Answer from the drawing. Dimensions are ordinates in mm from the lowest x, y and z of the part. Give positions to 0.01 mm unless a question says otherwise; leave off trailing zeros. Write each loop counter-clockwise with the first axis right and the second up, starting at its lowest first coordinate (ties: lowest second). Pieces come first, ordered by that corner, then holes. Notation, with made-up numbers: (76.5, -27.75) -> (132.5, -27.75) arc R30 cw to (132.5, 8.25) -> close; hole circle Ø4 at (-11.75, 70.25). An arc over 180 degrees is marked (long way). Use a Markdown table: item, result. Add a question column.
Q1. Consider line 1 (Y direction, x = 125.5, z = 1.05) (3 decimals); line 2 (X direction, y = 57, z = 2.9) (3 decimals). Determine where each line is inside the solid, lowest interval first.
Q2. Each of these flat-tipped pins is pushed along its axis until it touches: pin 1 Ø1 at (x, z) = (82, 2) entering from -Y (3 decimals); pin 2 Ø1 at (x, z) = (42.5, 1) entering from +Y; pin 3 Ø1 at (y, z) = (61, 2.5) entering from -X (3 decimals). Where does it stop, or does it pass through?
Q3. Section B-B, the plane x = 46 is taken. Give the vertices of the cut face in (y, z) (3 decimals), plus the area to 3 significant figures.
Q4. Section A-A, the plane y = 14.5 is taken. Give the vertices of the cut face in (x, z) (3 decimals).
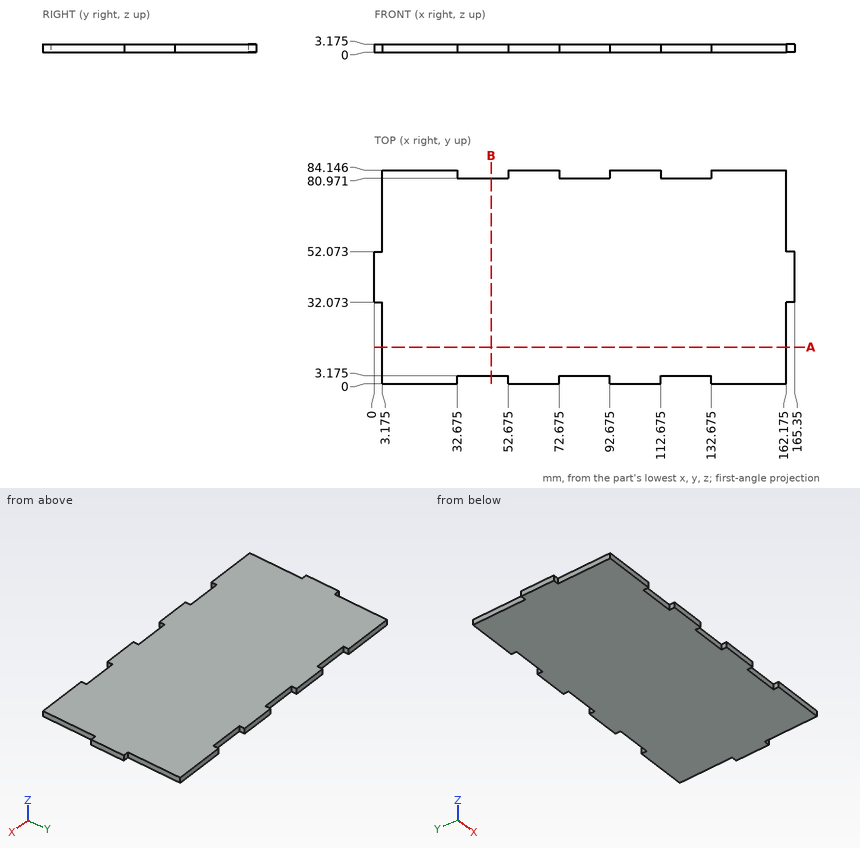
Result set:
| question | item | result |
|---|---|---|
| 1 | line 1 | y = 3.175 to 80.971 |
| 1 | line 2 | x = 3.175 to 162.175 |
| 2 | pin 1 | stops at y = 3.175 |
| 2 | pin 2 | stops at y = 80.97 |
| 2 | pin 3 | stops at x = 3.175 |
| 3 | outline | (3.175, 0) -> (80.971, 0) -> (80.971, 3.175) -> (3.175, 3.175) -> close |
| 3 | area | 247 mm2 |
| 4 | outline | (3.175, 0) -> (162.175, 0) -> (162.175, 3.175) -> (3.175, 3.175) -> close |
